CAD build for the part. Positions are in the model's coordinates, mm. Face numbers are marked on the shaded views. A direction names the side the tool comes from. Round coordinates to 2 decimals unless told otherwise and drop trailing zeros. Order: outer loops, then holes, each group sorted by start corner. A loop starts at its lowest first (then second) coordinate and runs counter-clockwise, first axis right, second up. Notation, with made-up numbers: (85.5, -0.75) - (126.5, -0.75) arc R8 ccw to (126.5, 9.25) - close; hole circle Ø5 at (-32, 71.25). An arc over 180 degrees is marked (long way). Write item = value, one per line.
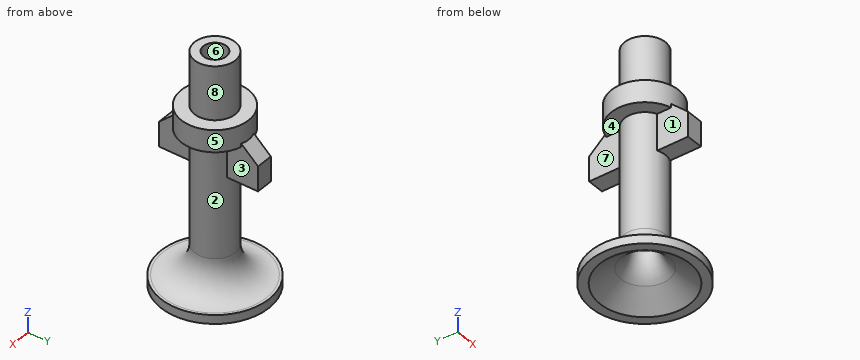
from build123d import *

# Parameters (mm, degrees)
BOSS_EXTRUDE1_DEPTH      = 0.95
BOSS_EXTRUDE1_DEPTH_BACK = 0.95


with BuildPart() as part:
    # Sketch1 → Revolve1 (revolve)
    with BuildSketch(Plane(origin=(0, 0, 0), x_dir=(0, 0, -1), z_dir=(1, 0, 0))):
        with BuildLine():
            Line((10.463274616, 2.3), (16.499380089, 2.3))
            Line((16.499380089, 2.3), (16.499380089, 3.8))
            Line((16.499380089, 3.8), (18.983450943, 3.8))
            Line((18.983450943, 3.8), (18.983450943, 2.3))
            Line((18.983450943, 2.3), (32, 2.3))
            ThreePointArc((32, 2.3), (34.474873734, 3.325126266), (35.5, 5.8))
            Line((35.5, 5.8), (35.5, 6.1))
            Line((35.5, 6.1), (36.5, 6.1))
            Line((36.5, 6.1), (36.5, 5.078211692))
            Line((36.5, 5.078211692), (34.771119215, 2.72674277))
            ThreePointArc((34.771119215, 2.72674277), (33.531386801, 1.676988608), (31.951260272, 1.3))
            Line((31.951260272, 1.3), (10.463274616, 1.3))
            Line((10.463274616, 1.3), (10.463274616, 2.3))
        make_face()
    revolve(axis=Axis((0, 0, -15.3), (0, 0, 1)))

    # Sketch2 → Boss-Extrude1 (add, two sides)
    with BuildSketch(Plane(origin=(0, 0, 0), x_dir=(0, 0, -1), z_dir=(1, 0, 0))) as boss_extrude1_sk:
        Polygon((23.1, 1.460737541), (23.1, 5.6), (20.3, 5.6), (16.583846242, 1.460737541), align=None)
        Polygon((16.583846242, -1.460737541), (23.1, -1.460737541), (23.1, -5.6), (20.3, -5.6), align=None)
    extrude(amount=BOSS_EXTRUDE1_DEPTH)
    extrude(boss_extrude1_sk.sketch, amount=-BOSS_EXTRUDE1_DEPTH_BACK)


solid = part.part
(1) Band-saw the part on A-A on y = 0. List the corners of the cut face in (x, z), plus the area to 3 significant figures.
Solved:
outline = (-6.1, -36.5) - (-5.08, -36.5) - (-2.73, -34.77) arc R3.5 ccw to (-1.3, -31.95) - (-1.3, -10.46) - (-2.3, -10.46) - (-2.3, -16.5) - (-3.8, -16.5) - (-3.8, -18.98) - (-2.3, -18.98) - (-2.3, -32) arc R3.5 cw to (-5.8, -35.5) - (-6.1, -35.5) - close; (1.3, -31.95) arc R3.5 ccw to (2.73, -34.77) - (5.08, -36.5) - (6.1, -36.5) - (6.1, -35.5) - (5.8, -35.5) arc R3.5 cw to (2.3, -32) - (2.3, -18.98) - (3.8, -18.98) - (3.8, -16.5) - (2.3, -16.5) - (2.3, -10.46) - (1.3, -10.46) - close
area = 61.0 mm²
(2) Band-saw the part on D-D on z = -14.75. List the corners of the cut face in (x, y).
Solved:
outline = circle Ø4.6 at (0, 0); hole circle Ø2.6 at (0, 0)
(3) Band-saw the part on B-B on z = -22.75. List the corners of the cut face in (x, y), plus the area to 3 significant figures.
Solved:
outline = (-0.95, -5.6) - (0.95, -5.6) - (0.95, -2.09) arc R2.3 ccw to (0.95, 2.09) - (0.95, 5.6) - (-0.95, 5.6) - (-0.95, 2.09) arc R2.3 ccw to (-0.95, -2.09) - close; hole circle Ø2.6 at (0, 0)
area = 24.1 mm²
(4) Drop flat-ended pins along their axis: pin 1 (1.5 mm diameter, centred on x = -0.5, y = 3.5, fed in from -Z); pin 2 (1.1 mm diameter, centred on y = 3.5, z = -20, fed in from +X); pin 3 (1 mm diameter, centred on x = 0.5, y = -4, fed in from -Z). Give the stop position or say it passes through.
Solved:
pin_1 = -35.92
pin_2 = 0.95
pin_3 = -36.1
(5) Probe line 1 along Y through (x, z) = (0, -15.5); line 2 along Y through (x, z) = (0, -21.5). List the from-to ranges inside material, lowest first.
Solved:
line_1 = -2.3 to -1.3, 1.3 to 2.3
line_2 = -5.6 to -1.3, 1.3 to 5.6
(6) Tool access for the marked faces 1, 2, 3, 4 and 5: list every direction of +Z, -Z, +X, -X, +Y, -Y with a clear straight run to the whole face (end or side of a thin tool).
Solved:
face_1 = -X, -Y
face_2 = none
face_3 = +X, +Y
face_4 = -X
face_5 = +Z
(7) Pull direction Y, two halves, no side cores. Call the marked faces 6, 7 and 8: released by +Y, released by -Y, zero draft, split by the parting line, or undercut.
Solved:
face_6 = undercut
face_7 = zero draft
face_8 = split by the parting line
